```python
from build123d import *

# Parameters (mm, degrees)
CROQUIS1_R                                           = 37.7
SALIENTE_EXTRUIR1_DEPTH                              = 7
REFRENTADO_PARA_TORNILLO_CON_CABEZA_TRON_D           = 3.4
REFRENTADO_PARA_TORNILLO_CON_CABEZA_TRON_CBORE_D     = 7
REFRENTADO_PARA_TORNILLO_CON_CABEZA_TRON_CBORE_DEPTH = 2.4
SALIENTE_EXTRUIR2_START                              = 13.1
CROQUIS4_R                                           = 37.7
CROQUIS4_R_2                                         = 32.8
SALIENTE_EXTRUIR2_DEPTH                              = 13.1
SALIENTE_EXTRUIR3_DEPTH                              = 10
REFRENTADO_PARA_TORNILLO_CON_CABEZA_2_D              = 3.4
REFRENTADO_PARA_TORNILLO_CON_CABEZA_2_CBORE_D        = 7
REFRENTADO_PARA_TORNILLO_CON_CABEZA_2_CBORE_DEPTH    = 2.4


with BuildPart() as part:
    # Croquis1 → Saliente-Extruir1 (new body)
    with BuildSketch(Plane.XY):
        Circle(CROQUIS1_R)
    extrude(amount=SALIENTE_EXTRUIR1_DEPTH)

    # Refrentado para tornillo con cabeza tron (through all)
    with Locations(Plane.XY.offset(7)):
        with Locations((0, 16), (13.856406461, 8), (13.856406461, -8), (0, -16), (-13.856406461, -8), (-13.856406461, 8)):
            CounterBoreHole(REFRENTADO_PARA_TORNILLO_CON_CABEZA_TRON_D / 2, REFRENTADO_PARA_TORNILLO_CON_CABEZA_TRON_CBORE_D / 2, REFRENTADO_PARA_TORNILLO_CON_CABEZA_TRON_CBORE_DEPTH)

    # Croquis4 → Saliente-Extruir2 (add)
    with BuildSketch(Plane(origin=(0, 0, 0), x_dir=(-1, 0, 0), z_dir=(0, 0, -1)).offset(SALIENTE_EXTRUIR2_START)):
        Circle(CROQUIS4_R)
        Circle(CROQUIS4_R_2, mode=Mode.SUBTRACT)
    extrude(amount=-SALIENTE_EXTRUIR2_DEPTH)

    # Croquis5 → Saliente-Extruir3 (add)
    with BuildSketch(Plane(origin=(0, 0, -13.1), x_dir=(-1, 0, 0), z_dir=(0, 0, -1))):
        with BuildLine():
            Line((-18.761663039, 32.7), (-100, 32.7))
            Line((-100, 32.7), (-100, -32.7))
            Line((-100, -32.7), (-18.761663039, -32.7))
            ThreePointArc((-18.761663039, -32.7), (-37.7, 0), (-18.761663039, 32.7))
        make_face()
    extrude(amount=-SALIENTE_EXTRUIR3_DEPTH)

    # Refrentado para tornillo con cabeza  2 (through all)
    with Locations(Plane.XY.offset(-3.1)):
        with Locations((75, 0), (90, 15), (60, -15), (60, 15), (90, -15)):
            CounterBoreHole(REFRENTADO_PARA_TORNILLO_CON_CABEZA_2_D / 2, REFRENTADO_PARA_TORNILLO_CON_CABEZA_2_CBORE_D / 2, REFRENTADO_PARA_TORNILLO_CON_CABEZA_2_CBORE_DEPTH)


solid = part.part
```
Design review of the part built by this model. Coordinates are the model's own, in mm. A direction names the side the tool comes from. Round coordinates to 2 decimals unless told otherwise and drop trailing zeros. Order: outer loops, then holes, each group sorted by start corner. A loop starts at its lowest first (then second) coordinate and runs counter-clockwise, first axis right, second up. Notation, with made-up numbers: (39.25, -18.75) - (73.25, -18.75) arc R13 ccw to (73.25, -7.75) - close; hole circle Ø1 at (-22.5, 34). An arc over 180 degrees is marked (long way). One line per question, with ' | ' between items.
Item 1: Take a section at A-A, the plane z = -11. Write out the cut boundary in (x, y), then the cut area to 3 significant figures.
Checks:
outline: (18.76, -32.7) - (100, -32.7) - (100, 32.7) - (18.76, 32.7) arc R37.7 ccw (long way) to start; hole circle Ø65.6 at (0, 0); hole circle Ø3.4 at (60, -15); hole circle Ø3.4 at (60, 15); hole circle Ø3.4 at (75, 0); hole circle Ø3.4 at (90, -15); hole circle Ø3.4 at (90, 15) | area: 5,470 mm²
Item 2: Take a section at C-C, the plane y = -21.5. Write out the cut boundary in (x, z), then the cut area to 3 significant figures.
Checks:
outline: (-30.97, -13.1) - (-24.77, -13.1) - (-24.77, 0) - (24.77, 0) - (24.77, -13.1) - (100, -13.1) - (100, -3.1) - (30.97, -3.1) - (30.97, 7) - (-30.97, 7) - close | area: 1,290 mm²
Item 3: Take a section at B-B, the plane x = 60. Write out the cut boundary in (y, z), then the cut area to 3 significant figures.
Checks:
outline: (-32.7, -13.1) - (-16.7, -13.1) - (-16.7, -5.5) - (-18.5, -5.5) - (-18.5, -3.1) - (-32.7, -3.1) - close; (-13.3, -13.1) - (13.3, -13.1) - (13.3, -5.5) - (11.5, -5.5) - (11.5, -3.1) - (-11.5, -3.1) - (-11.5, -5.5) - (-13.3, -5.5) - close; (16.7, -13.1) - (32.7, -13.1) - (32.7, -3.1) - (18.5, -3.1) - (18.5, -5.5) - (16.7, -5.5) - close | area: 569 mm²
Item 4: Take a section at D-D, the plane y = 8. Write out the cut boundary in (x, z), then the cut area to 3 significant figures.
Checks:
outline: (-36.84, -13.1) - (-31.81, -13.1) - (-31.81, 0) - (-15.56, 0) - (-15.56, 4.6) - (-17.36, 4.6) - (-17.36, 7) - (-36.84, 7) - close; (-12.16, 0) - (12.16, 0) - (12.16, 4.6) - (10.36, 4.6) - (10.36, 7) - (-10.36, 7) - (-10.36, 4.6) - (-12.16, 4.6) - close; (15.56, 0) - (31.81, 0) - (31.81, -13.1) - (100, -13.1) - (100, -3.1) - (36.84, -3.1) - (36.84, 7) - (17.36, 7) - (17.36, 4.6) - (15.56, 4.6) - close | area: 1,210 mm²
Item 5: Machinability: for faces 1 (the face through (14.078, 9.686, 2.268)), 2 (the face through (-12, -7, 4.6)), which of the approach directions +Z, -Z, +X, -X, +Y, -Y give a long, thin tool a straight path to every point of the face, cutting with its end or side? Answer none if there is none.
Checks:
face 1: +Z, -Z | face 2: +Z
Item 6: For P1, Ø4, axis at x = 52.5, z = -8.5, coming from the +Y side; P2, Ø5, axis at x = 42, z = -7.5, coming from the -Y side; P3, Ø4, axis at x = -13.86, y = -8, coming from the -Z side; P4, Ø7.5, axis at x = 14.5, y = 7.5, coming from the +Z side, all flat-tipped, find the tip position at first contact; note any pin that passes through.
Checks:
P1: y = 32.7 | P2: y = -32.7 | P3: z = 0 | P4: z = 7
Item 7: Wall thickness on line 1 (Y direction, x = 90, z = -5); line 2 (Y direction, x = 60, z = -10.5); line 3 (Z direction, x = 13.5, y = -22.5): over which ranges is each line inside the solid? List them lowest first. Write a range as [from, to].
Checks:
line 1: [-32.7, -18.5], [-11.5, 11.5], [18.5, 32.7] | line 2: [-32.7, -16.7], [-13.3, 13.3], [16.7, 32.7] | line 3: [0, 7]
